Work out the finished part from the listing and answer in its coordinate system (mm). Face numbers are marked on the shaded views. A direction names the side the tool comes from. Round coordinates to 2 decimals unless told otherwise and drop trailing zeros. Write each loop counter-clockwise with the first axis right and the second up, starting at its lowest first coordinate (ties: lowest second). Pieces come first, ordered by that corner, then holes.
1. Find section D-D (x = 25). Write down the section's boundary in (y, z), and give its area (3 significant figures).
2. Determine the mould class of the marked faces 5, 6, 7 and 8 for opening direction Y: pulls with the +Y half, pulls with the -Y half, needs draft (parallel to the pull), parting line crosses it, or undercut.
3. Find section C-C (y = 42.5). Write down the section's boundary in (x, z).
4. Straight lines are drawn through the part: probe 1 along Z at (x, y) = (8, 93); probe 2 along Y at (x, z) = (4.5, -31); probe 3 along Z at (x, y) = (36, -0.5). For each, find the intervals that lie inside material, in ascending order.
5. Find section A-A (z = 29.5). Write down the section's boundary in (x, y).
6. A tool of negligible diameter and unlimited length cuts with its end or side. For the marked faces 1, 2, 3 and 4, from which of +Z, -Z, +X, -X, +Y, -Y can it reach the whole face along a straight path? Write none if from no direction.
7. Flat-ended cylindrical pins translate along their axes: pin 1 Ø8 at (x, z) = (11.5, -41) entering from -Y; pin 2 Ø1.5 at (x, y) = (35, 5.5) entering from +Z; pin 3 Ø12 at (x, y) = (5, 13) entering from +Z. Find the tip coordinate at first contact, or state that the pin passes through.
8. Find section B-B (z = 0). Write down the section's boundary in (x, y).
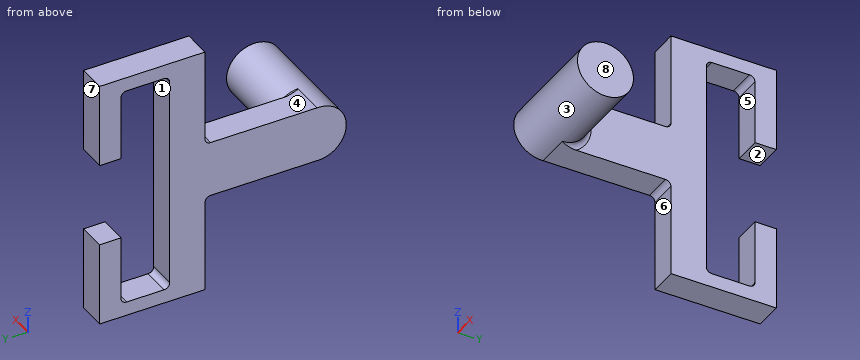
```python
from build123d import *

# Parameters (mm, degrees)
SKETCH2_R           = 12.7
BOSS_EXTRUDE1_DEPTH = 50.8
SKETCH3_W           = 25.4
SKETCH3_H           = 50.8
BOSS_EXTRUDE2_DEPTH = 12.7
SKETCH5_W           = 101.6
SKETCH5_H           = 16.002
BOSS_EXTRUDE3_DEPTH = 12.7
SKETCH6_W           = 6.35
SKETCH6_H           = 38.1
BOSS_EXTRUDE4_DEPTH = 12.7
SKETCH7_W           = 38.1
SKETCH7_H           = 9.652
BOSS_EXTRUDE5_DEPTH = 12.7
FILLET1_R           = 2.54


with BuildPart() as part:
    # Sketch2 → Boss-Extrude1 (new body)
    with BuildSketch(Plane(origin=(0, 0, 0), x_dir=(0, 0, -1), z_dir=(1, 0, 0))):
        Circle(SKETCH2_R)
    extrude(amount=BOSS_EXTRUDE1_DEPTH)

    # Sketch3 → Boss-Extrude2 (add)
    with BuildSketch(Plane.ZY):
        with Locations((0.014597196, 26.008732875)):
            Rectangle(SKETCH3_W, SKETCH3_H)
    extrude(amount=-BOSS_EXTRUDE2_DEPTH)


with BuildPart() as body_2:
    # Sketch5 → Boss-Extrude3 (new body)
    with BuildSketch(Plane(origin=(0, 0, 0), x_dir=(0, 0, -1), z_dir=(1, 0, 0))):
        with Locations((0, 59.392294155)):
            Rectangle(SKETCH5_W, SKETCH5_H)
    extrude(amount=BOSS_EXTRUDE3_DEPTH)

    # Sketch6 → Boss-Extrude4 (add)
    with BuildSketch(Plane(origin=(0, 0, 0), x_dir=(0, 0, -1), z_dir=(1, 0, 0))):
        with Locations((-53.975, 70.441294155)):
            Rectangle(SKETCH6_W, SKETCH6_H)
        with Locations((53.975, 70.441294155)):
            Rectangle(SKETCH6_W, SKETCH6_H)
    extrude(amount=BOSS_EXTRUDE4_DEPTH)

    # Sketch7 → Boss-Extrude5 (add)
    with BuildSketch(Plane(origin=(0, 0, 0), x_dir=(0, 0, -1), z_dir=(1, 0, 0))):
        with Locations((-38.1, 94.317294155)):
            Rectangle(SKETCH7_W, SKETCH7_H)
        with Locations((38.1, 94.317294155)):
            Rectangle(SKETCH7_W, SKETCH7_H)
    extrude(amount=BOSS_EXTRUDE5_DEPTH)


with BuildPart() as part_1:
    add(part.part)

    # Combine1: union body 2
    add(body_2.part)

    # Fillet1
    # the kernel refuses this fillet: 2.54 mm, written as the material it adds along each edge
    with BuildSketch(Plane(origin=(12.7, 51.391294155, 12.714597196), x_dir=(0, -1, 0), z_dir=(-1, 0, 0)), Plane(origin=(0, 51.391294155, -12.685402804), x_dir=(0, -1, 0), z_dir=(1, 0, 0)), Plane(origin=(0, 67.393294155, -50.8), x_dir=(0, 1, 0), z_dir=(1, 0, 0))) as fillet1_piece_1:
        with BuildLine():
            CenterArc((FILLET1_R, FILLET1_R), FILLET1_R, 180, 90)
            Line((0, FILLET1_R), (0, 0))
            Line((0, 0), (FILLET1_R, 0))
        make_face()
    extrude(amount=12.7)
    with BuildSketch(Plane(origin=(12.7, 0, 0), x_dir=(0, -0.4374901189408423, 0.8992232180216032), z_dir=(0, -0.8992232180216032, -0.4374901189408423))) as fillet1_piece_2_section:
        with BuildLine():
            CenterArc((12.7 + FILLET1_R, -FILLET1_R), FILLET1_R, 90, 90)
            Line((12.7 + FILLET1_R, 0), (12.7, 0))
            Line((12.7, 0), (12.7, -FILLET1_R))
        make_face()
    fillet1_piece_2 = revolve(axis=Axis((12.7, 0, 0), (-1, 0, 0)), revolution_arc=231.887700359, mode=Mode.PRIVATE)
    fillet1_piece_2 = split(fillet1_piece_2, bisect_by=Plane(origin=(13.416714054, 13.416714034, -12.685402804), z_dir=(0, 0, 1)), keep=Keep.TOP, mode=Mode.PRIVATE)
    fillet1_piece_2 = split(fillet1_piece_2, bisect_by=Plane(origin=(13.416714054, 0.608732875, 0.00073746), z_dir=(0, 1, 0)), keep=Keep.TOP, mode=Mode.PRIVATE)
    fillet1_piece_2 = split(fillet1_piece_2, bisect_by=Plane(origin=(13.416714054, 13.416714034, 12.714597196), z_dir=(0, 0, -1)), keep=Keep.TOP, mode=Mode.PRIVATE)
    add(fillet1_piece_2)
    with BuildSketch(Plane(origin=(0, 89.491294155, -50.8), x_dir=(0, -1, 0), z_dir=(1, 0, 0)), Plane(origin=(0, 89.491294155, 50.8), x_dir=(0, 0, -1), z_dir=(1, 0, 0)), Plane(origin=(0, 67.393294155, 50.8), x_dir=(0, 1, 0), z_dir=(1, 0, 0))) as fillet1_piece_3:
        with BuildLine():
            CenterArc((FILLET1_R, -FILLET1_R), FILLET1_R, 90, 90)
            Line((0, -FILLET1_R), (0, 0))
            Line((0, 0), (FILLET1_R, 0))
        make_face()
    extrude(amount=12.7)


solid = part_1.part
```
Worked answers:
1. outline: circle Ø25.4 at (0, 0)
1. area: 507 mm2
2. face 5: undercut
2. face 6: pulls with the -Y half
2. face 7: pulls with the +Y half
2. face 8: needs draft
3. outline: (0, -12.69) - (12.7, -12.69) - (12.7, 12.71) - (0, 12.71) - close
4. probe 1: z = -57.15 to -19.05, 19.05 to 57.15
4. probe 2: y = 51.39 to 67.39, 89.49 to 99.14
4. probe 3: z = -12.69 to 12.69
5. outline: (0, 51.39) - (12.7, 51.39) - (12.7, 67.39) - (0, 67.39) - close; (0, 89.49) - (12.7, 89.49) - (12.7, 99.14) - (0, 99.14) - close
6. face 1: +X, -X
6. face 2: +X, -X, +Y
6. face 3: +X
6. face 4: +Z, +X, -X, -Y
7. pin 1: stops at y = 51.39
7. pin 2: stops at z = 11.78
7. pin 3: stops at z = 12.71
8. outline: (0, -12.7) - (50.8, -12.7) - (50.8, 12.7) - (15.24, 12.7) arc R2.54 cw to (12.7, 15.24) - (12.7, 67.39) - (0, 67.39) - close
